```python
from build123d import *

# Parameters (mm, degrees)
SKETCH1_W           = 92.6
SKETCH1_H           = 300
BOSS_EXTRUDE1_DEPTH = 3
SKETCH2_R           = 2.25
SKETCH2_W           = 8.48
SKETCH2_H           = 51.5
SKETCH2_H_2         = 50
SKETCH2_H_3         = 53
CUT_EXTRUDE1_DEPTH  = 10
FILLET1_R           = 2
CUT_EXTRUDE3_DEPTH  = 8.5
SKETCH5_R           = 1.85
CUT_EXTRUDE4_DEPTH  = 10
SKETCH6_R           = 1.85
CUT_EXTRUDE5_DEPTH  = 10


with BuildPart() as part:
    # Sketch1 → Boss-Extrude1 (new body)
    with BuildSketch(Plane.XY):
        Rectangle(SKETCH1_W, SKETCH1_H)
    extrude(amount=BOSS_EXTRUDE1_DEPTH)

    # Sketch2 → Cut-Extrude1 (cut)
    with BuildSketch(Plane.XY):
        with Locations((-42.06, 75)):
            Circle(SKETCH2_R)
        with Locations((42.06, 125)):
            Circle(SKETCH2_R)
        with Locations((42.06, 25)):
            Circle(SKETCH2_R)
        with Locations((42.06, -75)):
            Circle(SKETCH2_R)
        with Locations((-42.06, -25)):
            Circle(SKETCH2_R)
        with Locations((-42.06, -125)):
            Circle(SKETCH2_R)
        with Locations((-42.06, 124.25)):
            Rectangle(SKETCH2_W, SKETCH2_H)
        with Locations((42.06, 75)):
            Rectangle(SKETCH2_W, SKETCH2_H_2)
        with Locations((42.06, -25)):
            Rectangle(SKETCH2_W, SKETCH2_H_2)
        with Locations((-42.06, 25)):
            Rectangle(SKETCH2_W, SKETCH2_H_3)
        with Locations((-42.06, -75)):
            Rectangle(SKETCH2_W, SKETCH2_H_3)
        with Locations((42.06, -125)):
            Rectangle(SKETCH2_W, SKETCH2_H_2)
    extrude(amount=CUT_EXTRUDE1_DEPTH, mode=Mode.SUBTRACT)

    # Fillet1
    fillet1_edges = [part.edges().sort_by_distance(p)[0] for p in [
        (46.3, -100, 1.5),
        (37.82, -100, 1.5),
        (37.82, -150, 1.5),
        (46.3, 50, 1.5),
        (46.3, 100, 1.5),
        (37.82, 100, 1.5),
        (37.82, 50, 1.5),
        (-46.3, -48.5, 1.5),
        (-46.3, -101.5, 1.5),
        (-37.82, -101.5, 1.5),
        (-37.82, -48.5, 1.5),
        (37.82, 0, 1.5),
        (37.82, -50, 1.5),
        (46.3, -50, 1.5),
        (46.3, 0, 1.5),
        (46.3, 150, 1.5),
        (-46.3, 51.5, 1.5),
        (-46.3, -150, 1.5),
        (-46.3, -1.5, 1.5),
        (-37.82, -1.5, 1.5),
        (-37.82, 51.5, 1.5),
        (-46.3, 98.5, 1.5),
        (-37.82, 98.5, 1.5),
        (-37.82, 150, 1.5),
    ]]
    fillet(fillet1_edges, radius=FILLET1_R)

    # Sketch4 → Cut-Extrude3 (cut)
    with BuildSketch(Plane(origin=(0, 0, 0), x_dir=(-1, 0, 0), z_dir=(0, 0, -1))):
        with BuildLine():
            Line((20, 90), (-20, 90))
            ThreePointArc((-20, 90), (-27.071067812, 92.928932188), (-30, 100))
            Line((-30, 100), (-30, 125))
            ThreePointArc((-30, 125), (-27.071067812, 132.071067812), (-20, 135))
            Line((-20, 135), (20, 135))
            ThreePointArc((20, 135), (27.071067812, 132.071067812), (30, 125))
            Line((30, 125), (30, 100))
            ThreePointArc((30, 100), (27.071067812, 92.928932188), (20, 90))
        make_face()
        with BuildLine():
            Line((25, -143), (-25, -143))
            ThreePointArc((-25, -143), (-28.535533906, -141.535533906), (-30, -138))
            Line((-30, -138), (-30, -98))
            ThreePointArc((-30, -98), (-28.535533906, -94.464466094), (-25, -93))
            Line((-25, -93), (25, -93))
            ThreePointArc((25, -93), (28.535533906, -94.464466094), (30, -98))
            Line((30, -98), (30, -138))
            ThreePointArc((30, -138), (28.535533906, -141.535533906), (25, -143))
        make_face()
    extrude(amount=-CUT_EXTRUDE3_DEPTH, mode=Mode.SUBTRACT)

    # Sketch5 → Cut-Extrude4 (cut)
    with BuildSketch(Plane(origin=(0, 0, 0), x_dir=(-1, 0, 0), z_dir=(0, 0, -1))):
        with Locations((0, 77.2)):
            Circle(SKETCH5_R)
        with Locations((-16.25, 47)):
            Circle(SKETCH5_R)
    extrude(amount=-CUT_EXTRUDE4_DEPTH, mode=Mode.SUBTRACT)

    # Sketch6 → Cut-Extrude5 (cut)
    with BuildSketch(Plane(origin=(0, 0, 0), x_dir=(-1, 0, 0), z_dir=(0, 0, -1))):
        with Locations((-4.5, 142.75)):
            Circle(SKETCH6_R)
        with Locations((10.5, 142.75)):
            Circle(SKETCH6_R)
    extrude(amount=-CUT_EXTRUDE5_DEPTH, mode=Mode.SUBTRACT)


solid = part.part
```
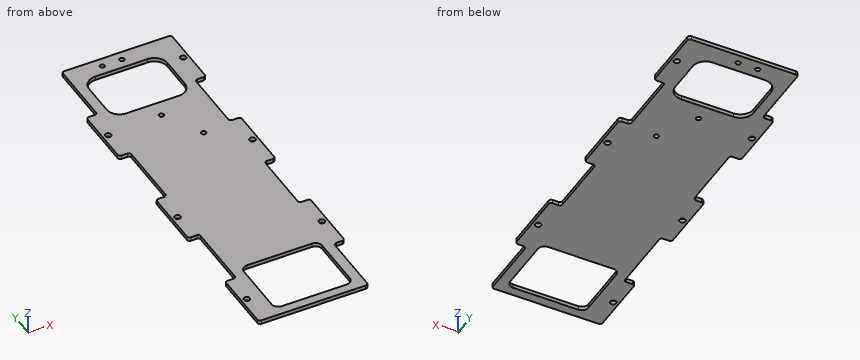
Check sheet for the modelled part. Datum: model origin and axes. Units: mm. Round coordinates to 2 decimals unless told otherwise and drop trailing zeros. Write each loop counter-clockwise with the first axis right and the second up, starting at its lowest first coordinate (ties: lowest second). Pieces come first, ordered by that corner, then holes. Notation, with made-up numbers: M 33.25,44.25 L 71.25,44.25 A21 ccw 71.25,60.25 Z; hole C 53.5,-28.5 d4. An arc over 180 degrees is marked long. Write item = value, one per line. Start each with the question number.
1. Section check A-A, the plane y = -115. Record the cut outline in (x, z).
2. Scan lines: line 1 (Y direction, x = -13.5, z = 2.05); line 2 (Y direction, x = 4.5, z = 0.9); line 3 (X direction, y = 142.75, z = 2.2). Record each from-to range of solid material in increasing order. Write a range as [from, to].
3. Section check B-B, the plane z = 2.2. State how many separate pieces and enclosed holes the cut face has, then the cut area to 3 significant figures.
4. Gauge pin test, flat ends, axial feed: pin 1 (1.5 mm diameter, centred on x = 43, z = 2, fed in from -Y); pin 2 (1 mm diameter, centred on y = 21.5, z = 1, fed in from -X). Record the tip position at first contact, or that the pin passes through.
Results found:
q1.outline = M -46.3,0 L -30,0 L -30,3 L -46.3,3 Z; M 30,0 L 37.82,0 L 37.82,3 L 30,3 Z
q2.line_1 = [-150, -143], [-93, 90], [135, 150]
q2.line_2 = [-150, -143], [-93, 90], [135, 140.9], [144.6, 150]
q2.line_3 = [-37.82, -12.35], [-8.65, 2.65], [6.35, 46.3]
q3.separate_pieces = 1
q3.enclosed_holes = 12
q3.area = 19,400 mm^2
q4.pin_1 = -100
q4.pin_2 = -37.82
